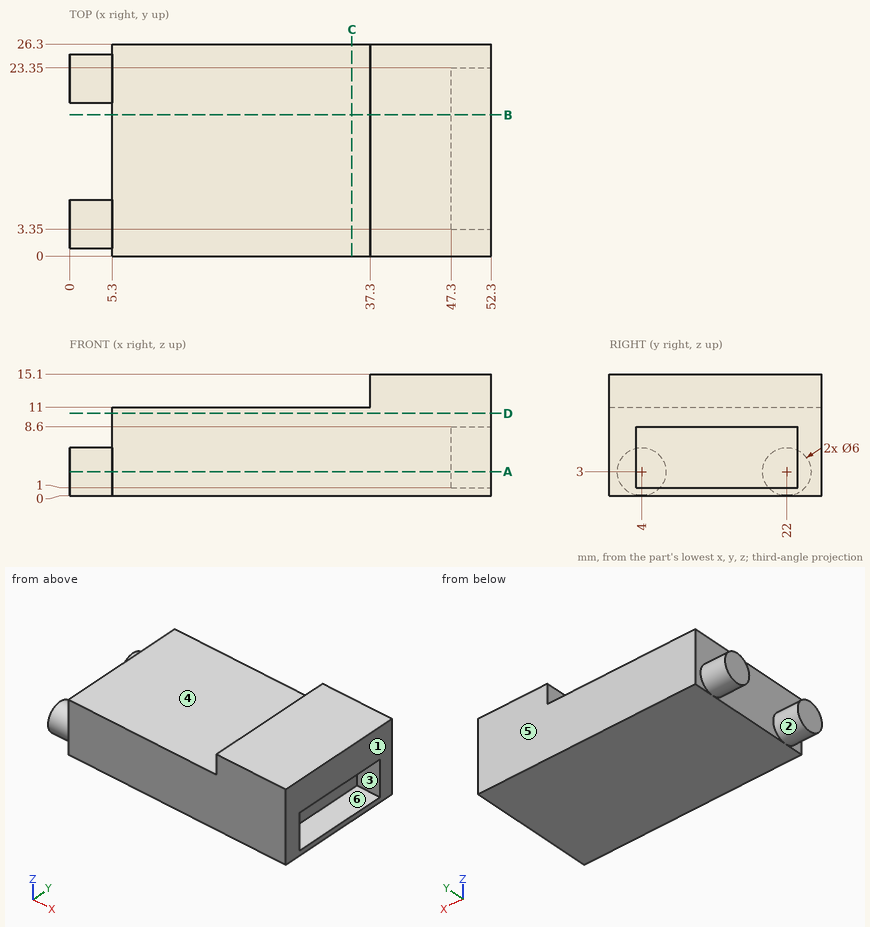
Check sheet for the drawn part. Datum: minimum x, y, z corner. Units: mm. A direction names the side the tool comes from. Coordinates: 2 decimals unless noted, no trailing zeros. Order: outer loops, then holes, each group sorted by start corner. A loop starts at its lowest first (then second) coordinate and runs counter-clockwise, first axis right, second up. Notation, with made-up numbers: (-1, 16) - (43, 16) arc R8 cw to (43, 21) - close; hole circle Ø4 at (24, -19). An arc over 180 degrees is marked (long way). Return JSON: item names as keys, results as strings.
(1) Section check B-B, the plane y = 17.5. Record the cut outline in (x, z).
Filled sheet:
{"outline": "(5.3, 0) - (52.3, 0) - (52.3, 1) - (47.3, 1) - (47.3, 8.6) - (52.3, 8.6) - (52.3, 15.1) - (37.3, 15.1) - (37.3, 11) - (5.3, 11) - close"}
(2) Mould release check, pull along Y, two halves, no side actions. Record for the marked faces 4, 5 and 6: pulls with the +Y half, pulls with the -Y half, needs draft (parallel to the pull), parting line crosses it, or undercut.
Filled sheet:
{"face 4": "needs draft", "face 5": "pulls with the +Y half", "face 6": "undercut"}
(3) Thickness scan on line 1 along Z through (x, y) = (48, 15.25); line 2 along X through (y, z) = (11.5, 10); line 3 along Y through (x, z) = (48.5, 5.25). Record the ranges inside material, lowest first.
Filled sheet:
{"line 1": "z = 0 to 1, 8.6 to 15.1", "line 2": "x = 5.3 to 52.3", "line 3": "y = 0 to 3.35, 23.35 to 26.3"}
(4) Go/stop test with flat-tipped pins: pin 1 (5.5 mm diameter, centred on y = 15.5, z = 5.5, fed in from -X); pin 2 (2 mm diameter, centred on y = 7.5, z = 12.5, fed in from -X); pin 3 (5 mm diameter, centred on x = 27.5, y = 13.5, fed in from +Z). Record where each tip stops, or that it passes through.
Filled sheet:
{"pin 1": "stops at x = 5.3", "pin 2": "stops at x = 37.3", "pin 3": "stops at z = 11"}
(5) Section check A-A, the plane z = 3. Record the cut outline in (x, y).
Filled sheet:
{"outline": "(0, 1) - (5.3, 1) - (5.3, 0) - (52.3, 0) - (52.3, 3.35) - (47.3, 3.35) - (47.3, 23.35) - (52.3, 23.35) - (52.3, 26.3) - (5.3, 26.3) - (5.3, 25) - (0, 25) - (0, 19) - (5.3, 19) - (5.3, 7) - (0, 7) - close"}
(6) Section check C-C, the plane x = 35. Record the cut outline in (y, z).
Filled sheet:
{"outline": "(0, 0) - (26.3, 0) - (26.3, 11) - (0, 11) - close"}
(7) Section check D-D, the plane z = 10.25. Record the cut outline in (x, y).
Filled sheet:
{"outline": "(5.3, 0) - (52.3, 0) - (52.3, 26.3) - (5.3, 26.3) - close"}
(8) Access from +Z, -Z, +X, -X, +Y, -Y to the whole of each face (thin tool, end or side, straight path). Record for the marked faces 1, 2 and 3.
Filled sheet:
{"face 1": "+Z, -Z, +X, +Y, -Y", "face 2": "-X", "face 3": "+X"}
